For this review, take the finished solid that the model builds, in its own axes (mm). A direction names the side the tool comes from. Round coordinates to 2 decimals unless told otherwise and drop trailing zeros. Write each loop counter-clockwise with the first axis right and the second up, starting at its lowest first coordinate (ties: lowest second). Pieces come first, ordered by that corner, then holes. Notation, with made-up numbers: (83.5, 20.25) - (103.5, 20.25) arc R29 ccw to (103.5, 57.25) - close; hole circle Ø6 at (-18.75, 76.25). An arc over 180 degrees is marked (long way). Answer in a Markdown table with one row per item. Add a question column.
from build123d import *

# Parameters (mm, degrees)
ESQUISSE2_W             = 3
ESQUISSE2_H             = 13.00905209
ENL_V_MAT_EXTRU_1_DEPTH = 4
ESQUISSE3_W             = 3
ESQUISSE3_H             = 13.12821898
ENL_V_MAT_EXTRU_2_DEPTH = 6


with BuildPart() as part:
    # Esquisse1 → Révolution2 (revolve)
    with BuildSketch(Plane.XY, mode=Mode.PRIVATE) as r_volution2_sk:
        with BuildLine():
            Line((-5, 1.5), (-5, 6))
            Line((-5, 6), (-8, 6))
            Line((-8, 6), (-8, 8))
            Line((-8, 8), (-5, 8))
            Line((-5, 8), (-5, 10.5))
            Line((-5, 10.5), (-6, 10.5))
            Line((-6, 10.5), (-6, 11))
            ThreePointArc((-6, 11), (-5.707106781, 11.707106781), (-5, 12))
            Line((-5, 12), (-3.5, 12))
            Line((-3.5, 12), (-3.5, 0))
            Line((-3.5, 0), (-5, 0))
            ThreePointArc((-5, 0), (-5.707106781, 0.292893219), (-6, 1))
            Line((-6, 1), (-6, 1.5))
            Line((-6, 1.5), (-5, 1.5))
        make_face()
    revolve(r_volution2_sk.sketch.rotate(Axis((0, 12, 0), (0, 1, 0)), 270), axis=Axis((0, 12, 0), (0, 1, 0)))

    # Esquisse2 → Enlèv. mat.-Extru.1 (cut)
    with BuildSketch(Plane(origin=(0, 12, 0), x_dir=(1, 0, 0), z_dir=(0, 1, 0))):
        with Locations((0.139511346, 0)):
            Rectangle(ESQUISSE2_W, ESQUISSE2_H)
    extrude(amount=-ENL_V_MAT_EXTRU_1_DEPTH, mode=Mode.SUBTRACT)

    # Esquisse3 → Enlèv. mat.-Extru.2 (cut)
    with BuildSketch(Plane.XZ):
        Rectangle(ESQUISSE3_W, ESQUISSE3_H)
    extrude(amount=-ENL_V_MAT_EXTRU_2_DEPTH, mode=Mode.SUBTRACT)


solid = part.part
Q1. Tool access review of faces 5 (the face through (-5.2, 10.5, 0.4)), 6 (the face through (-6, 10.8, -0.1)), 7 (the face through (5.3, 10.5, 0)): name each direction out of +Z, -Z, +X, -X, +Y, -Y from which nothing blocks a thin tool from reaching the whole face with its end or side.
Q2. Insertion check: pin 1 Ø1.3 at (y, z) = (3, 4.5) entering from +X; pin 2 Ø0.8 at (y, z) = (4.5, 5) entering from -X; pin 3 Ø1.5 at (y, z) = (8, -1.5) entering from -X; pin 4 Ø1 at (x, z) = (-1.5, -1) entering from +Y. Each pin has a flat end and moves straight along its axis. Give the tip position at first contact, or say it passes through.
Q3. Draft analysis for pull direction Y (two halves, no side actions). For faces 1 (the face through (-1.5, 3, 4)), 2 (the face through (4, 0, 0)), 3 (the face through (5, 9, 0)), 4 (the face through (-4, 12, 0)), state which applies: released by +Y, released by -Y, zero draft, split by the parting line, or undercut.
Q4. Add section B-B on x = 0. State the section outline as (y, z) points, then the cut area to 3 significant figures.
Q5. To check wall thickness, follow probe 1 along X at (y, z) = (9.5, 0); probe 2 along Y at (x, z) = (-2.5, -4.75); probe 3 along Y at (x, z) = (-4.5, -4.75). State the ranges of each line that lie inside material, in increasing order.
Q6. Add section C-C on y = 10.25. State the section outline as (x, z) points.
Q7. Add section D-D on x = 5.25. Count the separate pieces of the cut face and the enclosed holes in it, then the cut area to 3 significant figures.
Q8. Add section A-A on z = 0. State the section outline as (x, y) points, then the cut area to 3 significant figures.
Answer sheet:
| question | item | result |
|---|---|---|
| 1 | face 5 | -X |
| 1 | face 6 | -X, +Y |
| 1 | face 7 | +X |
| 2 | pin 1 | stops at x = 3.19 |
| 2 | pin 2 | stops at x = -1.96 |
| 2 | pin 3 | stops at x = -7.96 |
| 2 | pin 4 | passes through |
| 3 | face 1 | zero draft |
| 3 | face 2 | released by -Y |
| 3 | face 3 | undercut |
| 3 | face 4 | released by +Y |
| 4 | outline | (6, -8) - (8, -8) - (8, -3.5) - (6, -3.5) - close; (6, 3.5) - (8, 3.5) - (8, 8) - (6, 8) - close |
| 4 | area | 18.0 mm² |
| 5 | probe 1 | x = -5 to -3.5, 3.5 to 5 |
| 5 | probe 2 | y = 0.07 to 1.5, 6 to 8, 10.5 to 11.93 |
| 5 | probe 3 | y = 6 to 8 |
| 6 | outline | (-1.36, -4.81) - (-1.36, -3.22) arc R3.5 cw to (-1.36, 3.22) - (-1.36, 4.81) arc R5 ccw to start; (1.64, -4.72) arc R5 ccw to (1.64, 4.72) - (1.64, 3.09) arc R3.5 cw to (1.64, -3.09) - close |
| 7 | separate pieces | 3 |
| 7 | enclosed holes | 0 |
| 7 | area | 39.3 mm² |
| 8 | outline | (-8, 6) - (-5, 6) - (-5, 1.5) - (-6, 1.5) - (-6, 1) arc R1 ccw to (-5, 0) - (-3.5, 0) - (-3.5, 12) - (-5, 12) arc R1 ccw to (-6, 11) - (-6, 10.5) - (-5, 10.5) - (-5, 8) - (-8, 8) - close; (3.5, 0) - (5, 0) arc R1 ccw to (6, 1) - (6, 1.5) - (5, 1.5) - (5, 6) - (8, 6) - (8, 8) - (5, 8) - (5, 10.5) - (6, 10.5) - (6, 11) arc R1 ccw to (5, 12) - (3.5, 12) - close |
| 8 | area | 53.1 mm² |
